Autodesk Inventor part; units mm, degrees
ref_plane "GEH_XY" through (0, 0, 0) normal (1, 0, 0) x (0, 0, -1)
ref_plane "GEH_YZ" through (0, 0, 0) normal (0, 0, -1) x (0, 1, 0)
ref_plane "GEH_ZX" through (0, 0, 0) normal (0, 1, 0) x (1, 0, 0)
sketch "Sketch_1" plane through (0, 0, 0) normal (0, 0, 1) x (1, 0, 0)
  line L0 (10, 0) -> (0, 0)
  line L1 (0, 0) -> (0, 6)
  line L2 (0, 6) -> (2.5, 6)
  line L3 (2.5, 6) -> (2.5, 4)
  line L4 (2.5, 4) -> (7.4, 4)
  line L5 (7.4, 4) -> (8, 3.4)
  line L6 (8, 3.4) -> (8.5, 3.4)
  line L7 (8.5, 3.4) -> (8.5, 3.6)
  line L8 (8.5, 3.6) -> (8.8, 3.6)
  line L9 (8.8, 3.6) -> (9.9, 3.2)
  line L10 (9.9, 3.2) -> (10, 3.2)
  line L11 (10, 3.2) -> (10, 2.9)
  line L12 (10, 2.9) -> (5, 2.9)
  line L13 (5, 2.9) -> (5, 0)
  line L14 (5, 0) -> (0, 0)
revolve "Revolution1" add sketch "Sketch_1" angle 360 about axis through (10, 0, 0) along (1, 0, 0)
sketch "Sketch_2" plane through (0, 0, 0) normal (1, 0, 0) x (0, 1, 0)
  circle A0 centre (0, 0) radius 20
  line L0 (0, 5.7735) -> (-5, 2.8868)
  line L1 (-5, 2.8868) -> (-5, -2.8868)
  line L2 (-5, -2.8868) -> (0, -5.7735)
  line L3 (0, -5.7735) -> (5, -2.8868)
  line L4 (5, -2.8868) -> (5, 2.8868)
  line L5 (5, 2.8868) -> (0, 5.7735)
extrude "Extrusion1" cut sketch "Sketch_2" along normal blind 2.5
sketch "Sketch_3" plane through (0, 0, 1.7) normal (0, 0, 1) x (1, 0, 0)
  line L0 (9.8, 0.5) -> (5, 0.5)
  line L1 (5, 0.5) -> (5, 1)
  line L2 (5, 1) -> (9.3, 1)
  arc A0 (9.8, 0.5) -> (9.3, 1) centre (9.3, 0.5) ccw
  line L3 (9.8, 0.5) -> (5, 0.5)
revolve "Revolution2" add sketch "Sketch_3" angle 360 about axis through (9.8, 0.5, 1.7) along (1, 0, 0)
sketch "Pins_SKETCH_1" plane through (0, 0, -1.7) normal (0, 0, 1) x (1, 0, 0)
  line L0 (9.8, 0.5) -> (5, 0.5)
  line L1 (5, 0.5) -> (5, 1)
  line L2 (5, 1) -> (9.3, 1)
  arc A0 (9.8, 0.5) -> (9.3, 1) centre (9.3, 0.5) ccw
  line L3 (9.8, 0.5) -> (5, 0.5)
sketch "Pins_SKETCH_2" plane through (0, -1.95, -1.075) normal (0, 0, 1) x (1, 0, 0)
  line L0 (9.8, 0.5) -> (5, 0.5)
  line L1 (5, 0.5) -> (5, 1)
  line L2 (5, 1) -> (9.3, 1)
  arc A0 (9.8, 0.5) -> (9.3, 1) centre (9.3, 0.5) ccw
  line L3 (9.8, 0.5) -> (5, 0.5)
sketch "Pins_SKETCH_3" plane through (0, -1.95, 1.075) normal (0, 0, 1) x (1, 0, 0)
  line L0 (9.8, 0.5) -> (5, 0.5)
  line L1 (5, 0.5) -> (5, 1)
  line L2 (5, 1) -> (9.3, 1)
  arc A0 (9.8, 0.5) -> (9.3, 1) centre (9.3, 0.5) ccw
  line L3 (9.8, 0.5) -> (5, 0.5)
revolve "Revolution3" add sketch "Pins_SKETCH_1" angle 360 about axis through (9.8, 0.5, -1.7) along (1, 0, 0)
revolve "Revolution4" add sketch "Pins_SKETCH_2" angle 360 about axis through (9.8, -1.45, -1.075) along (1, 0, 0)
revolve "Revolution5" add sketch "Pins_SKETCH_3" angle 360 about axis through (9.8, -1.45, 1.075) along (1, 0, 0)
ref_plane "GEH_XY" through (0, 0, 0) normal (1, 0, 0) x (0, 0, -1)
ref_plane "GEH_YZ" through (0, 0, 0) normal (0, 0, -1) x (0, 1, 0)
ref_plane "GEH_ZX" through (0, 0, 0) normal (0, 1, 0) x (1, 0, 0)
properties part number "SCHUNK-SNT016581 Stecker EGP"
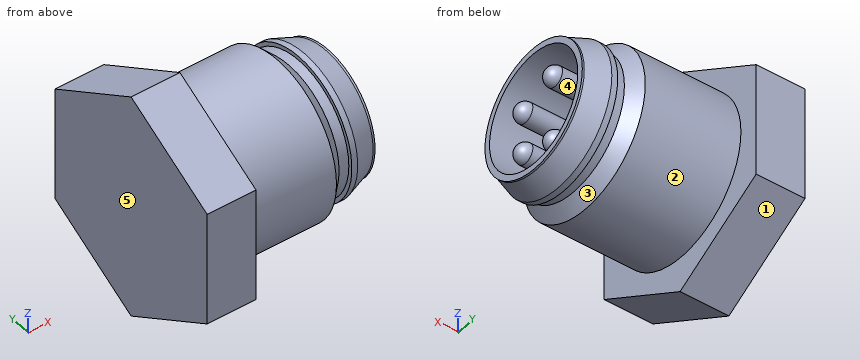
Work out the finished part from the listing and answer in its coordinate system (mm). Face numbers are marked on the shaded views. A direction names the side the tool comes from. Round coordinates to 2 decimals unless told otherwise and drop trailing zeros. Write each loop counter-clockwise with the first axis right and the second up, starting at its lowest first coordinate (ties: lowest second). Pieces come first, ordered by that corner, then holes. Notation, with made-up numbers: (17.25, -25) -> (63.25, -25) arc R18 cw to (63.25, -15) -> close; hole circle Ø4 at (50, 89.5). An arc over 180 degrees is marked (long way). Answer as CSV lines item,"result". Start each with the question number.
(1) The part is cut by section D-D, the plane z = 5.25. Give the vertices of the cut face in (x, y).
(2) Find the intervals of material crossed by probe 1 along Y at (x, z) = (7, -1); probe 2 along X at (y, z) = (-1.75, 4.25); probe 3 along Z at (x, y) = (9.25, -1.5), in increasing order.
(3) A tool of negligible diameter and unlimited length cuts with its end or side. For the marked faces 1 and 2, from which of +Z, -Z, +X, -X, +Y, -Y can it reach the whole face along a straight path? Write none if from no direction.
(4) Each of these flat-tipped pins is pushed along its axis until it touches: pin 1 (1.5 mm diameter, centred on x = 2.5, y = 2.5, fed in from -Z); pin 2 (1.5 mm diameter, centred on x = 5, y = 0, fed in from +Z); pin 3 (4 mm diameter, centred on x = 7.5, z = 3.5, fed in from -Y). Where does it stop, or does it pass through?
(5) The part is cut by section A-A, the plane x = 6. Give the vertices of the cut face in (y, z) (3 decimals), then the cut area to 3 significant figures.
(6) The part is cut by section B-B, the plane z = 0. Give the vertices of the cut face in (x, y), then the cut area to 3 significant figures.
(7) The mould has two halves that part along Y. Classify the marked faces 3, 4 and 5: +Y half, -Y half, draft (parallel to the pull), parting line (faces both ways), or undercut.
(8) The part is cut by section C-C, the plane x = 2.25. Give the vertices of the cut face in (y, z), then the cut area to 3 significant figures.
Output values:
1,outline,"(0, -0.91) -> (2.5, -0.91) -> (2.5, 0.91) -> (0, 0.91) -> close"
2,probe 1,"y = -3.87 to -2.72, -1.94 to -0.96, 2.72 to 3.87"
2,probe 2,"x = 0 to 2.5"
2,probe 3,"z = -3.09 to -2.48, -1.57 to -0.58, 0.58 to 1.57, 2.48 to 3.09"
3,face 1,"-Z, +X, -X, +Y"
3,face 2,"+X"
4,pin 1,"stops at z = -4.76"
4,pin 2,"stops at z = 4"
4,pin 3,"stops at y = -3.71"
5,outline,"circle Ø8 at (0, 0); circle Ø1 at (-1.45, -1.075); circle Ø1 at (-1.45, 1.075); circle Ø1 at (0.5, -1.7); circle Ø1 at (0.5, 1.7); hole circle Ø5.8 at (0, 0)"
5,area,"27.0 mm²"
6,outline,"(0, -5) -> (2.5, -5) -> (2.5, -4) -> (7.4, -4) -> (8, -3.4) -> (8.5, -3.4) -> (8.5, -3.6) -> (8.8, -3.6) -> (9.9, -3.2) -> (10, -3.2) -> (10, -2.9) -> (5, -2.9) -> (5, 2.9) -> (10, 2.9) -> (10, 3.2) -> (9.9, 3.2) -> (8.8, 3.6) -> (8.5, 3.6) -> (8.5, 3.4) -> (8, 3.4) -> (7.4, 4) -> (2.5, 4) -> (2.5, 5) -> (0, 5) -> close"
6,area,"53.3 mm²"
7,face 3,"parting line"
7,face 4,"undercut"
7,face 5,"draft"
8,outline,"(-5, -2.89) -> (0, -5.77) -> (5, -2.89) -> (5, 2.89) -> (0, 5.77) -> (-5, 2.89) -> close"
8,area,"86.6 mm²"
